Geometry: see drawing. Coordinates: mm, zero at the bounding-box minimum. Round coordinates to 2 decimals unless told otherwise and drop trailing zeros. Write each loop counter-clockwise with the first axis right and the second up, starting at its lowest first coordinate (ties: lowest second). Pieces come first, ordered by that corner, then holes.
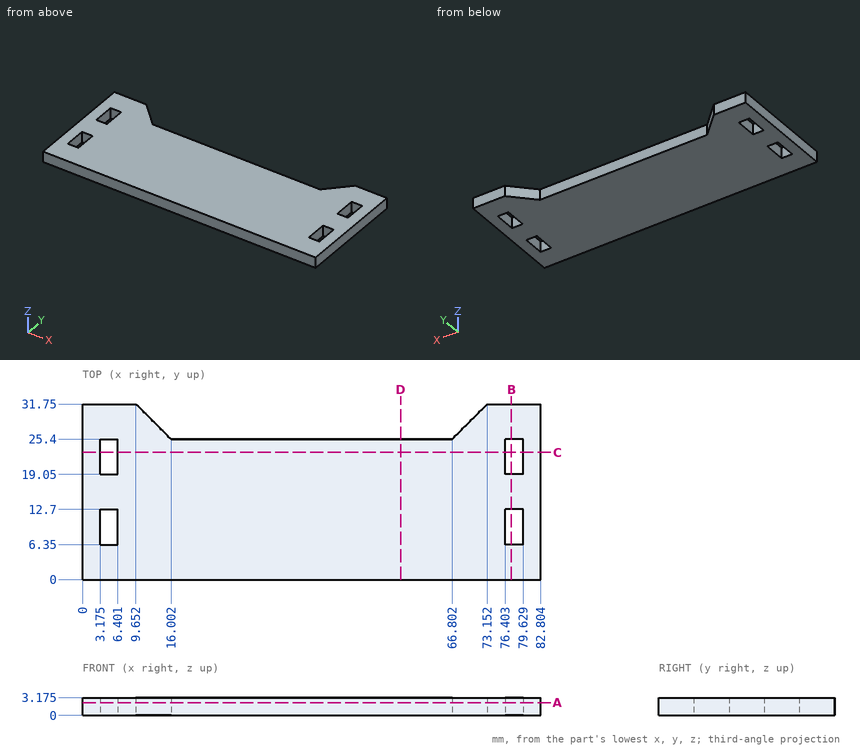
1) Section query D-D on x = 57.5. Return the cut outline in (y, z) (3 decimals).
Taken from the geometry:
outline: (0, 0) - (25.4, 0) - (25.4, 3.175) - (0, 3.175) - close
2) Section query A-A on z = 2.3. State how many separate pieces and enclosed holes the cut face has, then the cut area to 3 significant figures.
Taken from the geometry:
separate pieces: 1
enclosed holes: 4
area: 2,180 mm2
3) Section query C-C on y = 23. Return the cut outline in (x, z) (1 decimal), then the cut area to 3 significant figures.
Taken from the geometry:
outline: (0, 0) - (3.2, 0) - (3.2, 3.2) - (0, 3.2) - close; (6.4, 0) - (76.4, 0) - (76.4, 3.2) - (6.4, 3.2) - close; (79.6, 0) - (82.8, 0) - (82.8, 3.2) - (79.6, 3.2) - close
area: 242 mm2
4) Section query B-B on x = 77.5. Return the cut outline in (y, z) (3 decimals), then the cut area to 3 significant figures.
Taken from the geometry:
outline: (0, 0) - (6.35, 0) - (6.35, 3.175) - (0, 3.175) - close; (12.7, 0) - (19.05, 0) - (19.05, 3.175) - (12.7, 3.175) - close; (25.4, 0) - (31.75, 0) - (31.75, 3.175) - (25.4, 3.175) - close
area: 60.5 mm2
5) Material intervals for line 1 (X direction, y = 21.5, z = 1.1) (1 decimal); line 2 (Y direction, x = 5, z = 0.65); line 3 (Y direction, x = 38, z = 2.7), sorted ascending.
Taken from the geometry:
line 1: x = 0 to 3.2, 6.4 to 76.4, 79.6 to 82.8
line 2: y = 0 to 6.35, 12.7 to 19.05, 25.4 to 31.75
line 3: y = 0 to 25.4
